```python
from build123d import *

# Parameters (mm, degrees)
MODEL_R                 = 5
MODEL_W                 = 17.963611368
MODEL_H                 = 3.2
MODEL_W_2               = 17.963611367
SALIENTE_EXTRUIR1_DEPTH = 3


with BuildPart() as part:
    # Model → Saliente-Extruir1 (new body)
    with BuildSketch(Plane.XY):
        with BuildLine():
            Line((64.163611368, -39.615377633), (64.163611368, -4))
            Line((64.163611368, -4), (64.163611368, 15.5))
            Line((64.163611368, 15.5), (64.163611368, 34))
            ThreePointArc((64.163611368, 34), (64.456504586, 34.707106781), (65.163611368, 35))
            Line((65.163611368, 35), (71.836388632, 35))
            ThreePointArc((71.836388632, 35), (72.543495414, 35.292893219), (72.836388632, 36))
            Line((72.836388632, 36), (72.836388632, 54))
            ThreePointArc((72.836388632, 54), (73.129281851, 54.707106781), (73.836388632, 55))
            Line((73.836388632, 55), (134.836388632, 55))
            ThreePointArc((134.836388632, 55), (135.543495414, 54.707106781), (135.836388632, 54))
            Line((135.836388632, 54), (135.836388632, 36))
            ThreePointArc((135.836388632, 36), (136.129281851, 35.292893219), (136.836388632, 35))
            Line((136.836388632, 35), (144.836388632, 35))
            ThreePointArc((144.836388632, 35), (145.543495414, 34.707106781), (145.836388632, 34))
            Line((145.836388632, 34), (145.836388632, -94))
            ThreePointArc((145.836388632, -94), (145.543495414, -94.707106781), (144.836388632, -95))
            Line((144.836388632, -95), (65.163611368, -95))
            ThreePointArc((65.163611368, -95), (64.456504586, -94.707106781), (64.163611368, -94))
            Line((64.163611368, -94), (64.163611368, -39.615377633))
        make_face()
        with Locations((104.236388632, 6.8)):
            Circle(MODEL_R, mode=Mode.SUBTRACT)
        with Locations((118.418194316, 43.4)):
            Rectangle(MODEL_W, MODEL_H, mode=Mode.SUBTRACT)
        with Locations((90.254582949, 43.4)):
            Rectangle(MODEL_W_2, MODEL_H, mode=Mode.SUBTRACT)
    extrude(amount=SALIENTE_EXTRUIR1_DEPTH)


solid = part.part
```
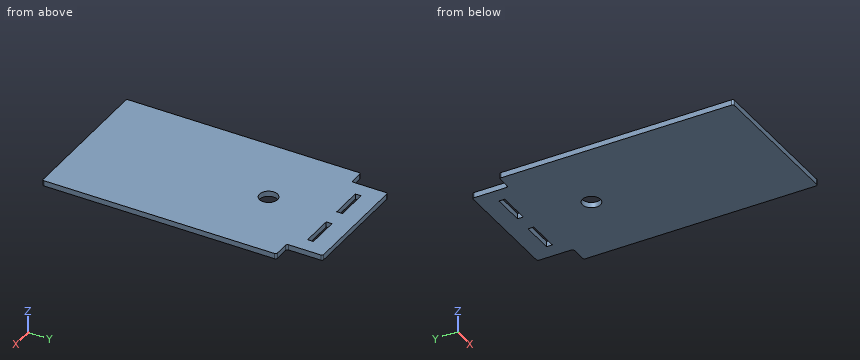
Geometry check sheet. Reference: the model listing, model coordinates, mm. Coordinates: 2 decimals unless noted, no trailing zeros. Order: outer loops, then holes, each group sorted by start corner. A loop starts at its lowest first (then second) coordinate and runs counter-clockwise, first axis right, second up.
Item 1: Scan lines: line 1 along Y through (x, z) = (115.5, 0.6); line 2 along Y through (x, z) = (139.5, 1.05); line 3 along X through (y, z) = (9, 1). Record each from-to range of solid material in increasing order.
Item 2: Section check B-B (z = 0.85). Enter the section's corners in (x, y).
Item 3: Depth check by flat-ended pin: pin 1 (0.9 mm diameter, centred on x = 68, z = 1.5, fed in from +Y); pin 2 (0.9 mm diameter, centred on y = 43.5, z = 1, fed in from +X); pin 3 (0.9 mm diameter, centred on y = 43.5, z = 1, fed in from -X). Enter the tip coordinate at first touch or a pass-through.
Item 4: Section check A-A (y = 6.8). Enter the section's corners in (x, z), plus the area to 3 significant figures.
Check sheet entries:
1. line 1: y = -95 to 41.8, 45 to 55
1. line 2: y = -95 to 35
1. line 3: x = 64.16 to 99.75, 108.73 to 145.84
2. outline: (64.16, -94) arc R1 ccw to (65.16, -95) - (144.84, -95) arc R1 ccw to (145.84, -94) - (145.84, 34) arc R1 ccw to (144.84, 35) - (136.84, 35) arc R1 cw to (135.84, 36) - (135.84, 54) arc R1 ccw to (134.84, 55) - (73.84, 55) arc R1 ccw to (72.84, 54) - (72.84, 36) arc R1 cw to (71.84, 35) - (65.16, 35) arc R1 ccw to (64.16, 34) - close; hole (81.27, 41.8) - (99.24, 41.8) - (99.24, 45) - (81.27, 45) - close; hole circle Ø10 at (104.24, 6.8); hole (109.44, 41.8) - (127.4, 41.8) - (127.4, 45) - (109.44, 45) - close
3. pin 1: stops at y = 35
3. pin 2: stops at x = 135.84
3. pin 3: stops at x = 72.84
4. outline: (64.16, 0) - (99.24, 0) - (99.24, 3) - (64.16, 3) - close; (109.24, 0) - (145.84, 0) - (145.84, 3) - (109.24, 3) - close
4. area: 215 mm2
